Can you work these out from the drawing? Everything is in mm from the part's minimum corner. A direction names the side the tool comes from. Coordinates: 2 decimals unless noted, no trailing zeros. Order: outer loops, then holes, each group sorted by start corner. A loop starts at its lowest first (then second) coordinate and runs counter-clockwise, first axis right, second up. Notation, with made-up numbers: (67.25, 81) - (76.25, 81) arc R27 ccw to (76.25, 119) - close; hole circle Ø5 at (-9, 11.5). An arc over 180 degrees is marked (long way). Use CSV: the item, a comma, the result in double quotes. Start each with the question number.
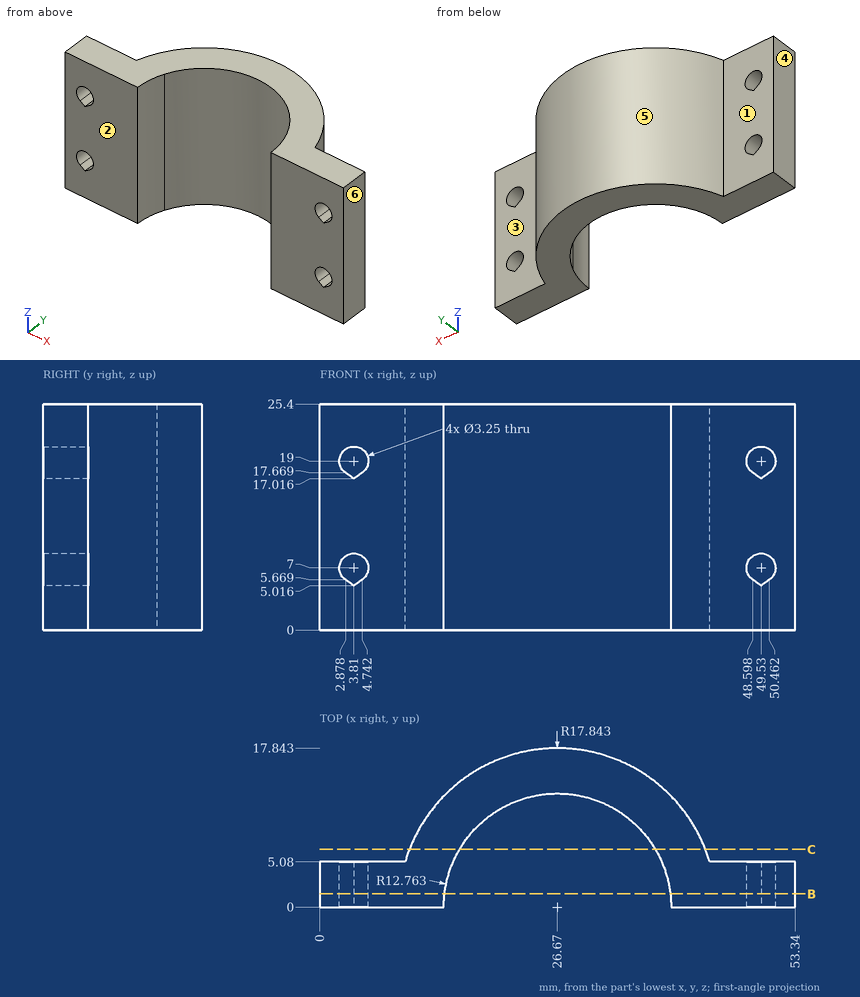
Item 1: Suppose I cut it at B-B on y = 1.5. State how many separate pieces and enclosed holes the cut face has, then the cut area to 3 significant figures.
Item 2: Suppose I cut it at C-C on y = 6.5. Write out the boundary of the cut face in (x, z) (1 decimal).
Item 3: For pin 1 Ø2 at (x, y) = (5.5, 5) entering from -Z; pin 2 Ø7.5 at (x, z) = (6.5, 7) entering from +Y (1 decimal); pin 3 Ø2.5 at (x, z) = (3.81, 7) entering from -Y; pin 4 Ø12 at (x, z) = (12.5, 15.5) entering from +Y, each with a flat end and sliding along its axis, tell me the tip position at first contact or that it passes through.
Item 4: For the marked faces 1 and 2, which set-ups out of +Z, -Z, +X, -X, +Y, -Y let a thin tool reach every point of the face, with its end or its side?
Item 5: We'd pull the mould along X, two halves only. Please class the marked faces 3, 4, 5 and 6: released by +X, released by -X, zero draft, split by the parting line, or undercut.
Item 6: Please list where these lines run through material, in increasing order: line 1 along Z through (x, y) = (49.53, 2.45) (1 decimal); line 2 along X through (y, z) = (2.5, 19) (1 decimal); line 3 along X through (y, z) = (2.7, 19) (1 decimal). Write a range as from..to.
Here are the results:
1,separate pieces,"2"
1,enclosed holes,"4"
1,area,"677 mm^2"
2,outline,"(10.1, 0) - (15.7, 0) - (15.7, 25.4) - (10.1, 25.4) - close; (37.7, 0) - (43.3, 0) - (43.3, 25.4) - (37.7, 25.4) - close"
3,pin 1,"z = 0"
3,pin 2,"y = 7"
3,pin 3,"through"
3,pin 4,"y = 15.86"
4,face 1,"+Z, -Z, -X, +Y"
4,face 2,"+Z, -Z, +X, -X, -Y"
5,face 3,"zero draft"
5,face 4,"released by -X"
5,face 5,"split by the parting line"
5,face 6,"released by +X"
6,line 1,"0..5, 8.6..17, 20.6..25.4"
6,line 2,"0..2.2, 5.4..14.2, 39.2..47.9, 51.2..53.3"
6,line 3,"0..2.2, 5.4..14.2, 39.1..47.9, 51.2..53.3"
